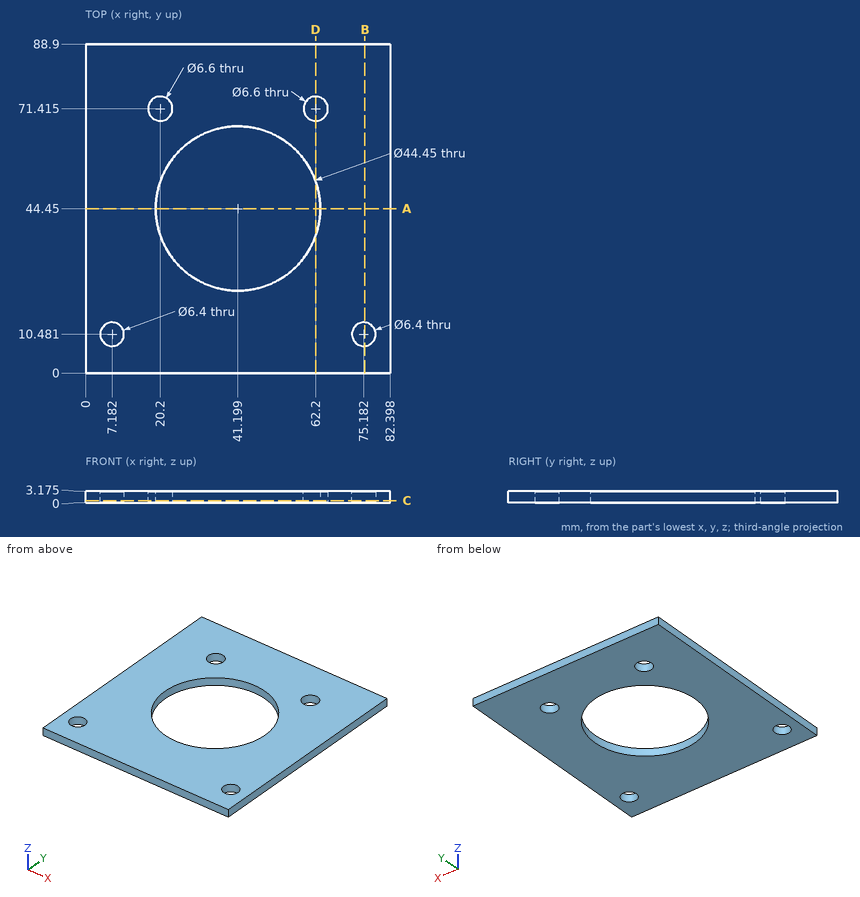
Input: dimensioned drawing with shaded views. Units: mm. Origin: part minimum x, y, z. Coordinates: 2 decimals unless noted, no trailing zeros. Write each loop counter-clockwise with the first axis right and the second up, starting at its lowest first coordinate (ties: lowest second). Pieces come first, ordered by that corner, then holes. Notation, with made-up numbers: (-22.75, 34) -> (-0.75, 34) arc R15 ccw to (-0.75, 62) -> close; hole circle Ø6 at (-5, -9). An arc over 180 degrees is marked (long way). Return JSON: item names as keys, results as strings. Group by question number.
1) Ray query, line 1 along X through (y, z) = (44.45, 2.4); line 2 along Y through (x, z) = (47, 1.25) (1 decimal); line 3 along X through (y, z) = (71, 0.4) (1 decimal). Return the intervals inside material, ascending.
2) Section query D-D, the plane x = 62.2. Return loops of the section in (y, z) (1 decimal).
3) Section query B-B, the plane x = 75.5. Return loops of the section in (y, z) (1 decimal).
4) Section query C-C, the plane z = 0.6. State how many separate pieces and enclosed holes the cut face has, plus the area to 3 significant figures.
5) Section query A-A, the plane y = 44.45. Return loops of the section in (x, z) (1 decimal).
6) Contact query for flat-ended pins moving along their axis: P1, Ø4, axis at x = 20.2, y = 71.42, coming from the +Z side; P2, Ø8.5, axis at x = 7.18, y = 10.48, coming from the -Z side. Output: stop coordinate, or through.
From the geometry:
{
 "1": {"line 1": "0 to 18.97, 63.42 to 82.4", "line 2": "0 to 23, 65.9 to 88.9", "line 3": "0 to 16.9, 23.5 to 58.9, 65.5 to 82.4"},
 "2": {"outline": "(0, 0) -> (37.2, 0) -> (37.2, 3.2) -> (0, 3.2) -> close; (51.7, 0) -> (68.1, 0) -> (68.1, 3.2) -> (51.7, 3.2) -> close; (74.7, 0) -> (88.9, 0) -> (88.9, 3.2) -> (74.7, 3.2) -> close"},
 "3": {"outline": "(0, 0) -> (7.3, 0) -> (7.3, 3.2) -> (0, 3.2) -> close; (13.7, 0) -> (88.9, 0) -> (88.9, 3.2) -> (13.7, 3.2) -> close"},
 "4": {"separate pieces": "1", "enclosed holes": "5", "area": "5,640 mm²"},
 "5": {"outline": "(0, 0) -> (19, 0) -> (19, 3.2) -> (0, 3.2) -> close; (63.4, 0) -> (82.4, 0) -> (82.4, 3.2) -> (63.4, 3.2) -> close"},
 "6": {"P1": "through", "P2": "z = 0"}
}
